The listing builds one solid part. Answer for the finished solid, in the listing's coordinates (mm). A direction names the side the tool comes from. Coordinates: 2 decimals unless noted, no trailing zeros. Loops run counter-clockwise (first coordinate to the right, second up) from the corner with the lowest first, then second, coordinate; pieces in that order, holes last. Notation, with made-up numbers: M -39.5,88 L -34.5,88 A30 ccw -34.5,111 Z; hole C 80,-11 d5. An arc over 180 degrees is marked long. Answer in a Markdown table with one row per item. Add a question column.
from build123d import *

# Parameters (mm, degrees)
SKETCH1_R           = 1.25
BOSS_EXTRUDE1_DEPTH = 3
SKETCH2_W           = 19
SKETCH2_H           = 10
BOSS_EXTRUDE2_DEPTH = 3
SKETCH3_R           = 2
CUT_EXTRUDE1_DEPTH  = 10
SKETCH4_W           = 2.95
SKETCH4_H           = 5.95
CUT_EXTRUDE2_DEPTH  = 33.182045836
FILLET1_R           = 5
SKETCH5_W           = 5.95
SKETCH5_H           = 2.95
BOSS_EXTRUDE3_DEPTH = 3
FILLET2_R           = 5
SKETCH6_R           = 7
CUT_EXTRUDE4_DEPTH  = 10


with BuildPart() as part:
    # Sketch1 → Boss-Extrude1 (new body)
    with BuildSketch(Plane.XY):
        with BuildLine():
            Line((7.5, 18.821590418), (9.5, 18.821590418))
            Line((9.5, 18.821590418), (9.5, 17.821590418))
            Line((9.5, 17.821590418), (7.5, 15.821590418))
            Line((7.5, 15.821590418), (7.5, 11.821590418))
            ThreePointArc((7.5, 11.821590418), (14, 0), (7.5, -11.821590418))
            Line((7.5, -11.821590418), (7.5, -15.821590418))
            Line((7.5, -15.821590418), (9.5, -17.821590418))
            Line((9.5, -17.821590418), (9.5, -18.821590418))
            Line((9.5, -18.821590418), (7.5, -18.821590418))
            Line((7.5, -18.821590418), (-7.5, -18.821590418))
            Line((-7.5, -18.821590418), (-9.5, -18.821590418))
            Line((-9.5, -18.821590418), (-9.5, -17.821590418))
            Line((-9.5, -17.821590418), (-7.5, -15.821590418))
            Line((-7.5, -15.821590418), (-7.5, -11.821590418))
            ThreePointArc((-7.5, -11.821590418), (-14, 0), (-7.5, 11.821590418))
            Line((-7.5, 11.821590418), (-7.5, 15.821590418))
            Line((-7.5, 15.821590418), (-9.5, 17.821590418))
            Line((-9.5, 17.821590418), (-9.5, 18.821590418))
            Line((-9.5, 18.821590418), (-7.5, 18.821590418))
            Line((-7.5, 18.821590418), (7.5, 18.821590418))
        make_face()
        with Locations((-10, 0)):
            Circle(SKETCH1_R, mode=Mode.SUBTRACT)
        with Locations((5, 8.660254038)):
            Circle(SKETCH1_R, mode=Mode.SUBTRACT)
        with Locations((5, -8.660254038)):
            Circle(SKETCH1_R, mode=Mode.SUBTRACT)
    extrude(amount=BOSS_EXTRUDE1_DEPTH)

    # Sketch2 → Boss-Extrude2 (add)
    with BuildSketch(Plane(origin=(0, 0, 0), x_dir=(-1, 0, 0), z_dir=(0, 0, -1))):
        with Locations((0, 23.821590418)):
            Rectangle(SKETCH2_W, SKETCH2_H)
        with Locations((0, -23.821590418)):
            Rectangle(SKETCH2_W, SKETCH2_H)
    extrude(amount=-BOSS_EXTRUDE2_DEPTH)

    # Sketch3 → Cut-Extrude1 (cut)
    with BuildSketch(Plane(origin=(0, 0, 0), x_dir=(-1, 0, 0), z_dir=(0, 0, -1))):
        Circle(SKETCH3_R)
    extrude(amount=-CUT_EXTRUDE1_DEPTH, mode=Mode.SUBTRACT)

    # Sketch4 → Cut-Extrude2 (cut, through all)
    with BuildSketch(Plane(origin=(0, 0, 0), x_dir=(-1, 0, 0), z_dir=(0, 0, -1))):
        with Locations((0, 21.796590418)):
            Rectangle(SKETCH4_W, SKETCH4_H)
        with Locations((0, -21.796590418)):
            Rectangle(SKETCH4_W, SKETCH4_H)
    extrude(amount=-CUT_EXTRUDE2_DEPTH, mode=Mode.SUBTRACT)

    # Fillet1
    fillet1_edges = [part.edges().sort_by_distance(p)[0] for p in [
        (9.5, -17.821590418, 1.5),
        (-9.5, -17.821590418, 1.5),
        (-9.5, 17.821590418, 1.5),
        (9.5, 17.821590418, 1.5),
        (-9.5, 28.821590418, 1.5),
        (9.5, 28.821590418, 1.5),
        (-9.5, -28.821590418, 1.5),
        (9.5, -28.821590418, 1.5),
    ]]
    fillet(fillet1_edges, radius=FILLET1_R)

    # Sketch5 → Boss-Extrude3 (add)
    # profile 1 of 2: a face of its own
    with BuildSketch(Plane(origin=(0, 0, 0), x_dir=(-1, 0, 0), z_dir=(0, 0, -1))):
        with BuildLine():
            Line((-12.412669938, -6.475), (-29.771590418, -6.475))
            Line((-29.771590418, -6.475), (-29.771590418, 6.475))
            Line((-29.771590418, 6.475), (-12.412669938, 6.475))
            ThreePointArc((-12.412669938, 6.475), (-14, 0), (-12.412669938, -6.475))
        make_face()
        with Locations((-21.796590418, 0)):
            Rectangle(SKETCH5_W, SKETCH5_H, mode=Mode.SUBTRACT)
    # profile 2 of 2: a face of its own
    with BuildSketch(Plane(origin=(0, 0, 0), x_dir=(-1, 0, 0), z_dir=(0, 0, -1))):
        with BuildLine():
            Line((29.771590418, 6.475), (12.412669938, 6.475))
            ThreePointArc((12.412669938, 6.475), (14, 0), (12.412669938, -6.475))
            Line((12.412669938, -6.475), (29.771590418, -6.475))
            Line((29.771590418, -6.475), (29.771590418, 6.475))
        make_face()
        with Locations((21.796590418, 0)):
            Rectangle(SKETCH5_W, SKETCH5_H, mode=Mode.SUBTRACT)
    extrude(amount=-BOSS_EXTRUDE3_DEPTH)

    # Fillet2
    fillet2_edges = [part.edges().sort_by_distance(p)[0] for p in [
        (-29.771590418, 6.475, 1.5),
        (-29.771590418, -6.475, 1.5),
        (29.771590418, -6.475, 1.5),
        (29.771590418, 6.475, 1.5),
    ]]
    fillet(fillet2_edges, radius=FILLET2_R)

    # Sketch6 → Cut-Extrude4 (cut)
    with BuildSketch(Plane.XY.offset(3)):
        with Locations((-7.346152109, 11.220655855)):
            Circle(SKETCH6_R)
    extrude(amount=-CUT_EXTRUDE4_DEPTH, mode=Mode.SUBTRACT)


solid = part.part
(1) A cutting plane is placed at B-B (x = 15). Give the vertices of the cut face in (y, z) (3 decimals).
(2) A cutting plane is placed at A-A (y = 0). Give the vertices of the cut face in (x, z), plus the area to 3 significant figures.
(3) Each of these flat-tipped pins is pushed along its axis until it touches: pin 1 (0.9 mm diameter, centred on y = -14.5, z = 2, fed in from +X); pin 2 (0.9 mm diameter, centred on x = 17, z = 2, fed in from +Y) (3 decimals); pin 3 (1.5 mm diameter, centred on x = -19, z = 1.5, fed in from -Y) (3 decimals). Where does it stop, or does it pass through?
(4) For faces 1 (the face through (-9.109, -17.954, 1.521)), 2 (the face through (10.274, 9.51, 1.479)), 3 (the face through (19, 6.475, 1)), determine the directions among +Z, -Z, +X, -X, +Y, -Y from which every point of the face is accessible in a straight line to the end or side of a thin tool.
(5) A cutting plane is placed at C-C (z = 2.5). State how many separate pieces and enclosed holes the cut face has, plus the area to 3 significant figures.
(6) The mould has two halves that part along Y. Classify faces 4 (the face through (-11.25, 0.05, 1.48)), 5 (the face through (-7.996, 27.396, 1.521)), 6 (the face through (-19, -6.475, 1)): released by +Y, released by -Y, zero draft, split by the parting line, or undercut.
(7) Straight lines are drawn through the part: line 1 (Y direction, x = 5, z = 0.9); line 2 (Y direction, x = 21.5, z = 1.65) (3 decimals); line 3 (Y direction, x = 16, z = 2.25) (3 decimals). For each, find the intervals that lie inside material, in ascending order.
(8) A cutting plane is placed at D-D (y = 14). Give the vertices of the cut face in (x, z).
Solved:
| question | item | result |
|---|---|---|
| 1 | outline | M -6.475,0 L 6.475,0 L 6.475,3 L -6.475,3 Z |
| 2 | outline | M -29.77,0 L -24.77,0 L -24.77,3 L -29.77,3 Z; M -18.82,0 L -11.25,0 L -11.25,3 L -18.82,3 Z; M -8.75,0 L -2,0 L -2,3 L -8.75,3 Z; M 2,0 L 18.82,0 L 18.82,3 L 2,3 Z; M 24.77,0 L 29.77,0 L 29.77,3 L 24.77,3 Z |
| 2 | area | 123 mm² |
| 3 | pin 1 | stops at x = 7.5 |
| 3 | pin 2 | stops at y = 6.475 |
| 3 | pin 3 | stops at y = -6.475 |
| 4 | face 1 | +Z, -Z, -X |
| 4 | face 2 | +Z, -Z, +X |
| 4 | face 3 | +Z, -Z, +X, +Y |
| 5 | separate pieces | 1 |
| 5 | enclosed holes | 8 |
| 5 | area | 1,350 mm² |
| 6 | face 4 | undercut |
| 6 | face 5 | released by +Y |
| 6 | face 6 | released by -Y |
| 7 | line 1 | y = -28.8 to -9.91, -7.41 to 7.41, 9.91 to 28.8 |
| 7 | line 2 | y = -6.475 to -1.475, 1.475 to 6.475 |
| 7 | line 3 | y = -6.475 to 6.475 |
| 8 | outline | M -0.92,0 L 7.5,0 L 7.5,3 L -0.92,3 Z |
